Geometry: final body of the model. Coordinates: model frame, mm. A direction names the side the tool comes from. Give positions to 0.01 mm unless a question says otherwise; leave off trailing zeros. Write each loop counter-clockwise with the first axis right and the second up, starting at its lowest first coordinate (ties: lowest second). Pieces come first, ordered by that corner, then holes. Notation, with made-up numbers: (17.25, 29.5) -> (73.25, 29.5) arc R7 ccw to (73.25, 35.5) -> close; hole circle Ø4 at (-16.75, -35). An arc over 180 degrees is marked (long way). Answer as a JSON object with one key per item and string values.
from build123d import *

# Parameters (mm, degrees)
SKETCH215_R             = 2.1
PAD110_DEPTH            = 15
POCKET079_DEPTH         = 42.3742142452
POCKET079_DEPTH_BACK    = 42.3742142452
POCKET115_DEPTH         = 3.001
POCKET115_DEPTH_BACK    = 3.001
BODY091_ROLL_ANGLE      = -180
BODY091_PLACEMENT_ANGLE = 90


with BuildPart() as part:
    # Sketch215 → Pad110 (new body)
    with BuildSketch(Plane.XY):
        with BuildLine():
            ThreePointArc((-8.25, 3), (-11.25, 0), (-8.25, -3))
            Line((0, -3), (-8.25, -3))
            Line((0, 3), (0, -3))
            Line((0, 3), (-8.25, 3))
        make_face()
        with Locations((-8.25, 0)):
            Circle(SKETCH215_R, mode=Mode.SUBTRACT)
    extrude(amount=PAD110_DEPTH)

    # Sketch216 → Pocket079 (cut, two sides)
    with BuildSketch(Plane.XZ) as pocket079_sk:
        with BuildLine():
            Line((-3.2536045714, 15), (-3.117150432, 7.1825475936))
            ThreePointArc((-3.117150432, 7.1825475936), (-2.8182120012, 6.4867495508), (-2.1173027369, 6.2))
            Line((0, 6.2), (-2.1173027369, 6.2))
            Line((0, 6.2), (0, 15))
            Line((-3.2536045714, 15), (0, 15))
        make_face()
    extrude(amount=-POCKET079_DEPTH, mode=Mode.SUBTRACT)
    extrude(pocket079_sk.sketch, amount=POCKET079_DEPTH_BACK, mode=Mode.SUBTRACT)

    # Sketch268 → Pocket115 (cut, two sides)
    with BuildSketch(Plane.XZ) as pocket115_sk:
        Polygon((-12, 8), (-5, 15), (-12, 15), align=None)
    extrude(amount=-POCKET115_DEPTH, mode=Mode.SUBTRACT)
    extrude(pocket115_sk.sketch, amount=POCKET115_DEPTH_BACK, mode=Mode.SUBTRACT)

    # Mirrored046: part across Sketch216 V_Axis


with BuildPart() as part_1:
    add(part.part)
    add(part.part.mirror(Plane(origin=(0, 0, 0), x_dir=(0, -1, 0), z_dir=(1, 0, 0))))


with BuildPart() as part_2:
    # Body091 roll: moved
    add(part_1.part.rotate(Axis((0, 0, 0), (1, 0, 0)), BODY091_ROLL_ANGLE))


with BuildPart() as part_3:
    # Body091 placement: moved
    add(part_2.part.moved(Location((71.5, 19.83, 20))).rotate(Axis((71.5, 19.83, 20), (0, 0, 1)), BODY091_PLACEMENT_ANGLE))


solid = part_3.part
Q1. Cut plane C-C (z = 9.5). Return the cut outline in (x, y), and give its area (3 significant figures).
Values:
{"outline": "(68.5, 11.58) arc R3 ccw to (68.77, 10.33) -> (69.81, 10.33) arc R2.1 cw (long way) to (73.19, 10.33) -> (74.23, 10.33) arc R3 ccw to (74.5, 11.58) -> (74.5, 16.65) -> (68.5, 16.65) -> close; (68.5, 23.01) -> (74.5, 23.01) -> (74.5, 28.08) arc R3 ccw to (74.23, 29.33) -> (73.19, 29.33) arc R2.1 cw (long way) to (69.81, 29.33) -> (68.77, 29.33) arc R3 ccw to (68.5, 28.08) -> close", "area": "51.8 mm²"}
Q2. First-contact query: P1, Ø2, axis at x = 71, y = 19, coming from the -Z side. Flat tip, straight axial feed; report the tip coordinate or a pass-through.
Values:
{"P1": "z = 13.8"}
Q3. Cut plane D-D (z = 12.25). Return the cut outline in (x, y).
Values:
{"outline": "(68.5, 11.58) arc R3 ccw to (74.5, 11.58) -> (74.5, 16.7) -> (68.5, 16.7) -> close; (68.5, 22.96) -> (74.5, 22.96) -> (74.5, 28.08) arc R3 ccw to (68.5, 28.08) -> close; hole circle Ø4.2 at (71.5, 11.58); hole circle Ø4.2 at (71.5, 28.08)"}
Q4. Set-up query: faces 1 (the flat face through (72, 16, 5)), 2 (the cylindrical face through (71.5, 17, 13.5)). Return all of +Z, -Z, +X, -X, +Y, -Y with unobstructed straight access to the full face (end or side cutting, diameter ignored); none if empty.
Values:
{"face 1": "-Z, +X, -X, +Y, -Y", "face 2": "-Z, +X, -X"}
Q5. Cut plane B-B (z = 19). Return the cut outline in (x, y).
Values:
{"outline": "(68.5, 11.58) arc R3 ccw to (74.5, 11.58) -> (74.5, 28.08) arc R3 ccw to (68.5, 28.08) -> close; hole circle Ø4.2 at (71.5, 11.58); hole circle Ø4.2 at (71.5, 28.08)"}
Q6. Cut plane A-A (x = 71.5). Return the cut outline in (y, z).
Values:
{"outline": "(8.58, 11.25) -> (9.48, 10.35) -> (9.48, 20) -> (8.58, 20) -> close; (13.68, 6.15) -> (14.83, 5) -> (16.58, 5) -> (16.71, 12.82) arc R1 cw to (17.71, 13.8) -> (21.95, 13.8) arc R1 cw to (22.95, 12.82) -> (23.08, 5) -> (24.83, 5) -> (25.98, 6.15) -> (25.98, 20) -> (13.68, 20) -> close; (30.18, 10.35) -> (31.08, 11.25) -> (31.08, 20) -> (30.18, 20) -> close"}
Q7. Material intervals for L1, parallel to Y at x = 71.5, z = 15.25; L2, parallel to X at y = 11.58, z = 9; L3, parallel to Y at x = 69.95, z = 16.75, sorted ascending. Write a range as from..to.
Values:
{"L1": "8.58..9.48, 13.68..25.98, 30.18..31.08", "L2": "68.5..69.4, 73.6..74.5", "L3": "9.01..10.16, 13..26.66, 29.5..30.65"}
Q8. Mould query, pull axis Y, two halves, no side actions, for faces 3 (the cylindrical face through (71.458, 22.656, 13.506)), 4 (the flat face through (72, 20, 20)), 5 (the cylindrical face through (71.57, 8.58, 15.51)), 6 (the cylindrical face through (72.131, 13.583, 14.711)). Classes: pulls with the +Y half, pulls with the -Y half, needs draft (parallel to the pull), parting line crosses it, or undercut.
Values:
{"face 3": "undercut", "face 4": "needs draft", "face 5": "pulls with the -Y half", "face 6": "undercut"}
